```python
from build123d import *

# Parameters (mm, degrees)
F0_R     = 15.24
F0_W     = 10.16
F0_H     = 10.16
F1_DEPTH = 8.89
F2_R     = 15.24
F3_DEPTH = 63.5
F4_R     = 1.27
F5_R     = 2.54


with BuildPart() as f1:
    # F0 (on Top) → F1 (new body)
    with BuildSketch(Plane.XY):
        Circle(F0_R)
        Rectangle(F0_W, F0_H, mode=Mode.SUBTRACT)
    extrude(amount=F1_DEPTH)

    # F2 (on face) → F3 (join)
    with BuildSketch(Plane.XY.offset(8.89)):
        Circle(F2_R)
        Polygon((-12.065, 0), (-6.0325, 10.448596), (6.0325, 10.448596), (12.065, 0), (6.0325, -10.448596), (-6.0325, -10.448596), align=None, mode=Mode.SUBTRACT)
    extrude(amount=F3_DEPTH)

    # F4
    f4_edges = [f1.edges().sort_by_distance(p)[0] for p in [
        (-5.08, -5.08, 4.445),
        (-5.08, 5.08, 4.445),
        (5.08, -5.08, 4.445),
        (5.08, 5.08, 4.445),
    ]]
    fillet(f4_edges, radius=F4_R)

    # F5
    f5_edges = [f1.edges().sort_by_distance(p)[0] for p in [
        (-15.24, 0, 0),
        (-15.24, 0, 72.39),
    ]]
    fillet(f5_edges, radius=F5_R)


solid = f1.part
```
Could you check a few things on this model? Use its own coordinates, in mm. A direction names the side the tool comes from. Give positions to 0.01 mm unless a question says otherwise; leave off trailing zeros. Write each loop counter-clockwise with the first axis right and the second up, starting at its lowest first coordinate (ties: lowest second). Pieces come first, ordered by that corner, then holes. Notation, with made-up numbers: (-18.5, 77.5) -> (39.5, 77.5) arc R34 cw to (39.5, 108.5) -> close; hole circle Ø6 at (58.5, 43.5). An arc over 180 degrees is marked (long way). Write each question's results on one line, items separated by ' | '.
1. On a 3-axis mill with a long thin cutter (end or side, diameter ignored), from which of +Z, -Z, +X, -X, +Y, -Y can I reach the whole of each face in a straight line? I mean faces 1 (the flat face through (0, -10.449, 40)), 2 (the cylindrical face through (-4.718, 4.698, 4.507)), 3 (the flat face through (-9.5, 4.8, 72.39)). Say none if no direction works.
Check sheet entries:
face 1: +Z | face 2: +Z, -Z | face 3: +Z, +X, -X, +Y, -Y
2. I need wall thicknesses on L1, parallel to Z at x = 7, y = -8.5; L2, parallel to Y at x = -9, z = 46; L3, parallel to Y at x = 1.5, z = 29.5. Which ranges of each line are inside material? Lowest first, please.
Check sheet entries:
L1: z = 0 to 8.89 | L2: y = -12.3 to -5.31, 5.31 to 12.3 | L3: y = -15.17 to -10.45, 10.45 to 15.17
3. Will these pins go through, and if not, where does the flat tip stop? pin 1 Ø8 at (y, z) = (-9.5, 22.5) entering from +X; pin 2 Ø1.5 at (y, z) = (-9.5, 38.5) entering from -X; pin 3 Ø4 at (x, z) = (-9.5, 19) entering from -Y.
Check sheet entries:
pin 1: stops at x = 14.21 | pin 2: stops at x = -12.48 | pin 3: stops at y = -13.27
4. I want a section at B-B, the plane z = 18. Write out the boundary of the cut face in (x, y) (1 decimal).
Check sheet entries:
outline: circle Ø30.5 at (0, 0); hole (-12.1, 0) -> (-6, -10.4) -> (6, -10.4) -> (12.1, 0) -> (6, 10.4) -> (-6, 10.4) -> close
5. If we mould it in two halves opening along Y, with no side actions, what happens to faces 4 (the flat face through (5.5, 0.2, 0)), 5 (the cylindrical face through (-3.3, -14.88, 35.72)), 6 (the flat face through (-9.09, 5.15, 40.2))? For each: released by +Y, released by -Y, zero draft, split by the parting line, or undercut.
Check sheet entries:
face 4: zero draft | face 5: split by the parting line | face 6: undercut
6. I want a section at A-A, the plane x = 0. Write out the boundary of the cut face in (y, z), then the cut area to 3 significant figures.
Check sheet entries:
outline: (-15.24, 2.54) arc R2.54 ccw to (-12.7, 0) -> (-5.08, 0) -> (-5.08, 8.89) -> (-10.45, 8.89) -> (-10.45, 72.39) -> (-12.7, 72.39) arc R2.54 ccw to (-15.24, 69.85) -> close; (5.08, 0) -> (12.7, 0) arc R2.54 ccw to (15.24, 2.54) -> (15.24, 69.85) arc R2.54 ccw to (12.7, 72.39) -> (10.45, 72.39) -> (10.45, 8.89) -> (5.08, 8.89) -> close | area: 784 mm²
